Geometry check sheet. Reference: the model listing, model coordinates, mm. Give positions to 0.01 mm unless a question says otherwise; leave off trailing zeros. Write each loop counter-clockwise with the first axis right and the second up, starting at its lowest first coordinate (ties: lowest second). Pieces come first, ordered by that corner, then holes. Notation, with made-up numbers: M 2.25,11 L 22.25,11 A21 cw 22.25,37 Z; hole C 1.5,-4.5 d4. An arc over 180 degrees is marked long. Use one line per item in the form item = value. Start each with the question number.
```python
from build123d import *

# Parameters (mm, degrees)
EXTRUDE_1_DEPTH     = 5
SKETCH_2_R          = 1.6
SKETCH_2_W          = 7.5
SKETCH_2_H          = 3.1
CUT_EXTRUDE_1_DEPTH = 5
EXTRUDE_START       = -2.5
SKETCH_3_R          = 2.6
EXTRUDE_2_DEPTH     = 2.5
EXTRUDE_START_2     = 15
SKETCH_4_W          = 20
SKETCH_4_H          = 20
EXTRUDE_3_DEPTH     = 15
CUT_EXTRUDE_2_REACH = 135.15
SKETCH_5_R          = 1.55
FILLET_2_R          = 3


with BuildPart() as part:
    # 草图1 → 凸台-拉伸1 (new body)
    with BuildSketch(Plane.XY):
        with BuildLine():
            Line((0, 0), (45, 0))
            Line((45, 0), (45, 113.1))
            ThreePointArc((45, 113.1), (22.5, 152.07114317), (0, 113.1))
            Line((0, 113.1), (0, 0))
        make_face()
        with BuildLine():
            Line((19.44, 129.02), (25.56, 129.02))
            ThreePointArc((25.56, 129.02), (22.5, 138.2), (19.44, 129.02))
        make_face(mode=Mode.SUBTRACT)
    extrude(amount=EXTRUDE_1_DEPTH)

    # 草图2 → 切除-拉伸1 (cut)
    with BuildSketch(Plane.XY.offset(5)):
        with Locations((40, 8.1)):
            Circle(SKETCH_2_R)
        with Locations((5, 8.1)):
            Circle(SKETCH_2_R)
        with Locations((31.25, 1.55)):
            Rectangle(SKETCH_2_W, SKETCH_2_H)
        with Locations((13.75, 1.55)):
            Rectangle(SKETCH_2_W, SKETCH_2_H)
        Polygon((7.5, 26), (2.303847577, 23), (2.303847577, 17), (7.5, 14), (12.696152423, 17), (12.696152423, 23), align=None)
        Polygon((22.5, 26), (17.303847577, 23), (17.303847577, 17), (22.5, 14), (27.696152423, 17), (27.696152423, 23), align=None)
        Polygon((37.5, 26), (32.303847577, 23), (32.303847577, 17), (37.5, 14), (42.696152423, 17), (42.696152423, 23), align=None)
        Polygon((15, 56), (9.803847577, 53), (9.803847577, 47), (15, 44), (20.196152423, 47), (20.196152423, 53), align=None)
        Polygon((15, 36), (9.803847577, 33), (9.803847577, 27), (15, 24), (20.196152423, 27), (20.196152423, 33), align=None)
        Polygon((30, 36), (24.803847577, 33), (24.803847577, 27), (30, 24), (35.196152423, 27), (35.196152423, 33), align=None)
        Polygon((30, 56), (24.803847577, 53), (24.803847577, 47), (30, 44), (35.196152423, 47), (35.196152423, 53), align=None)
        Polygon((37.5, 46), (32.303847577, 43), (32.303847577, 37), (37.5, 34), (42.696152423, 37), (42.696152423, 43), align=None)
        Polygon((22.5, 46), (17.303847577, 43), (17.303847577, 37), (22.5, 34), (27.696152423, 37), (27.696152423, 43), align=None)
        Polygon((7.5, 46), (2.303847577, 43), (2.303847577, 37), (7.5, 34), (12.696152423, 37), (12.696152423, 43), align=None)
        Polygon((15, 76), (9.803847577, 73), (9.803847577, 67), (15, 64), (20.196152423, 67), (20.196152423, 73), align=None)
        Polygon((30, 76), (24.803847577, 73), (24.803847577, 67), (30, 64), (35.196152423, 67), (35.196152423, 73), align=None)
        Polygon((37.5, 66), (32.303847577, 63), (32.303847577, 57), (37.5, 54), (42.696152423, 57), (42.696152423, 63), align=None)
        Polygon((22.5, 66), (17.303847577, 63), (17.303847577, 57), (22.5, 54), (27.696152423, 57), (27.696152423, 63), align=None)
        Polygon((7.5, 66), (2.303847577, 63), (2.303847577, 57), (7.5, 54), (12.696152423, 57), (12.696152423, 63), align=None)
        Polygon((15, 96), (9.803847577, 93), (9.803847577, 87), (15, 84), (20.196152423, 87), (20.196152423, 93), align=None)
        Polygon((30, 96), (24.803847577, 93), (24.803847577, 87), (30, 84), (35.196152423, 87), (35.196152423, 93), align=None)
        Polygon((37.5, 86), (32.303847577, 83), (32.303847577, 77), (37.5, 74), (42.696152423, 77), (42.696152423, 83), align=None)
        Polygon((22.5, 86), (17.303847577, 83), (17.303847577, 77), (22.5, 74), (27.696152423, 77), (27.696152423, 83), align=None)
        Polygon((7.5, 86), (2.303847577, 83), (2.303847577, 77), (7.5, 74), (12.696152423, 77), (12.696152423, 83), align=None)
        Polygon((15, 116), (9.803847577, 113), (9.803847577, 107), (15, 104), (20.196152423, 107), (20.196152423, 113), align=None)
        Polygon((30, 116), (24.803847577, 113), (24.803847577, 107), (30, 104), (35.196152423, 107), (35.196152423, 113), align=None)
        Polygon((37.5, 106), (32.303847577, 103), (32.303847577, 97), (37.5, 94), (42.696152423, 97), (42.696152423, 103), align=None)
        Polygon((22.5, 106), (17.303847577, 103), (17.303847577, 97), (22.5, 94), (27.696152423, 97), (27.696152423, 103), align=None)
        Polygon((7.5, 106), (2.303847577, 103), (2.303847577, 97), (7.5, 94), (12.696152423, 97), (12.696152423, 103), align=None)
    extrude(amount=-CUT_EXTRUDE_1_DEPTH, mode=Mode.SUBTRACT)

    # 草图3 → 凸台-拉伸2 (add)
    with BuildSketch(Plane.XY.offset(5).offset(EXTRUDE_START)):
        with BuildLine():
            Line((19.44, 129.02), (25.56, 129.02))
            ThreePointArc((25.56, 129.02), (22.5, 138.2), (19.44, 129.02))
        make_face()
        with Locations((22.5, 133.1)):
            Circle(SKETCH_3_R, mode=Mode.SUBTRACT)
    extrude(amount=EXTRUDE_2_DEPTH)

    # 草图4 → 凸台-拉伸3 (add)
    with BuildSketch(Plane(origin=(0, 0, 0), x_dir=(-1, 0, 0), z_dir=(0, 0, -1)).offset(EXTRUDE_START_2)):
        with Locations((-22.5, 133.1)):
            Rectangle(SKETCH_4_W, SKETCH_4_H)
        with BuildLine():
            Line((-25.56, 129.02), (-19.44, 129.02))
            ThreePointArc((-19.44, 129.02), (-22.5, 138.2), (-25.56, 129.02))
        make_face(mode=Mode.SUBTRACT)
    extrude(amount=-EXTRUDE_3_DEPTH)

    # 切除-拉伸2: up to this face of the body (flat: up to its plane)
    cut_extrude_2_end = Plane(part.part.faces().sort_by_distance((22.5, 143.1, -7.5))[0])
    # 草图5 → 切除-拉伸2 (cut, up to the picked face)
    with BuildSketch(Plane.XZ.offset(-123.1), mode=Mode.PRIVATE) as cut_extrude_2_sk1:
        with Locations(Location((22.5, -7.5, 0), (0, 0, 270))):
            Circle(SKETCH_5_R)
    cut_extrude_2_tool1 = split(extrude(cut_extrude_2_sk1.sketch, amount=-CUT_EXTRUDE_2_REACH, mode=Mode.PRIVATE), bisect_by=cut_extrude_2_end, keep=Keep.BOTH, mode=Mode.PRIVATE)
    add(cut_extrude_2_tool1.solids().sort_by(Axis((22.5, 123.1, -7.5), (0, 1, 0)))[0], mode=Mode.SUBTRACT)

    # 圆角2
    fillet_2_edges = [part.edges().sort_by_distance(p)[0] for p in [
        (32.5, 133.1, 0),
        (32.5, 143.1, -7.5),
        (22.5, 123.1, 0),
        (32.5, 123.1, -7.5),
        (12.5, 133.1, 0),
        (12.5, 123.1, -7.5),
        (22.5, 143.1, 0),
        (12.5, 143.1, -7.5),
    ]]
    fillet(fillet_2_edges, radius=FILLET_2_R)


solid = part.part
```
(1) Sectioned sample at C-C, the plane y = 8.1. Record the boundary of the cut face in (x, z), plus the area to 3 significant figures.
(2) Sectioned sample at B-B, the plane x = 5. Record the boundary of the cut face in (y, z), plus the area to 3 significant figures.
(3) Thickness scan on probe 1 along X at (y, z) = (126.85, -7.5); probe 2 along Z at (x, y) = (36, 47.5); probe 3 along X at (y, z) = (125, -2.75). Record the ranges inside material, lowest first. Write a range as [from, to].
(4) Draft check along Y on faces 1 (the flat face through (12.5, 133, -9)), 2 (the flat face through (24.804, 30, 3)). Enter one of: released by +Y, released by -Y, zero draft, split by the parting line, or undercut.
(5) Sectioned sample at A-A, the plane y = 61.5. Record the boundary of the cut face in (x, z).
(6) Depth check by flat-ended pin: pin 1 (2.5 mm diameter, centred on y = 78.5, z = 1.5, fed in from +X); pin 2 (3 mm diameter, centred on x = 23.5, y = 134, fed in from -Z); pin 3 (4 mm diameter, centred on y = 39, z = 1.5, fed in from -X). Enter the tip coordinate at first touch or a pass-through.
(7) Sectioned sample at D-D, the plane z = -11.75. Record the boundary of the cut face in (x, y).
Numbers:
q1.outline = M 0,0 L 3.4,0 L 3.4,5 L 0,5 Z; M 6.6,0 L 38.4,0 L 38.4,5 L 6.6,5 Z; M 41.6,0 L 45,0 L 45,5 L 41.6,5 Z
q1.area = 193 mm2
q2.outline = M 0,0 L 6.5,0 L 6.5,5 L 0,5 Z; M 9.7,0 L 15.44,0 L 15.44,5 L 9.7,5 Z; M 24.56,0 L 35.44,0 L 35.44,5 L 24.56,5 Z; M 44.56,0 L 55.44,0 L 55.44,5 L 44.56,5 Z; M 64.56,0 L 75.44,0 L 75.44,5 L 64.56,5 Z; M 84.56,0 L 95.44,0 L 95.44,5 L 84.56,5 Z; M 104.56,0 L 145.29,0 L 145.29,5 L 104.56,5 Z
q2.area = 483 mm2
q3.probe_1 = [12.5, 20.95], [24.05, 32.5]
q3.probe_2 = [0, 5]
q3.probe_3 = [12.7, 32.3]
q4.face_1 = zero draft
q4.face_2 = undercut
q5.outline = M 0,0 L 2.3,0 L 2.3,5 L 0,5 Z; M 12.7,0 L 17.3,0 L 17.3,5 L 12.7,5 Z; M 27.7,0 L 32.3,0 L 32.3,5 L 27.7,5 Z; M 42.7,0 L 45,0 L 45,5 L 42.7,5 Z
q6.pin_1 = 45
q6.pin_2 = 2.5
q6.pin_3 = 0
q7.outline = M 12.5,126.1 A3 ccw 15.5,123.1 L 29.5,123.1 A3 ccw 32.5,126.1 L 32.5,140.1 A3 ccw 29.5,143.1 L 15.5,143.1 A3 ccw 12.5,140.1 Z; hole M 19.44,129.02 L 25.56,129.02 A5.1 ccw long Z
